Check sheet for the modelled part. Datum: model origin and axes. Units: mm. Round coordinates to 2 decimals unless told otherwise and drop trailing zeros. Loops run counter-clockwise (first coordinate to the right, second up) from the corner with the lowest first, then second, coordinate; pieces in that order, holes last. Notation, with made-up numbers: (44.25, 58.5) - (87.25, 58.5) arc R8 ccw to (87.25, 69.5) - close; hole circle Ø6 at (79, 53). An arc over 180 degrees is marked (long way). Answer in a Markdown table with one row per item. Add a question column.
(1) Cross-section at A-A on z = -25. Enter the section's corners in (x, y), then the cut area to 3 significant figures.
(2) Gauge pin test, flat end, axial feed: pin 1 (3 mm diameter, centred on x = -0.5, z = -481.5, fed in from +Y). Record the tip position at first contact, or that the pin passes through.
(3) Thickness scan on line 1 along X through (y, z) = (3.25, -240); line 2 along X through (y, z) = (6, -360); line 3 along Z through (x, y) = (-8, -3.5). Record the ranges inside material, lowest first.
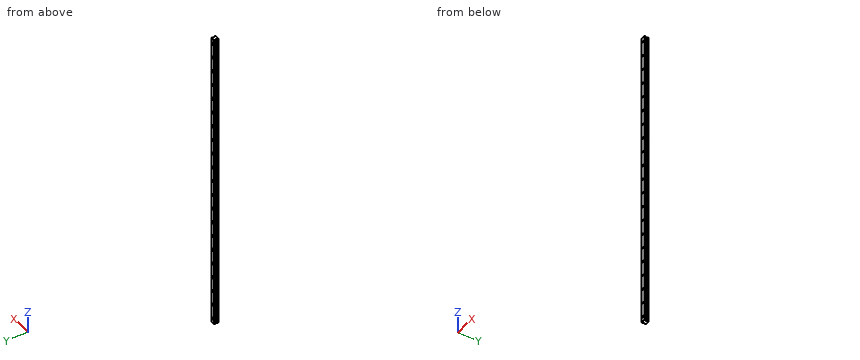
from build123d import *

# Parameters (mm, degrees)
BOSS_EXTRUDE1_DEPTH      = 620
BOSS_EXTRUDE1_DEPTH_BACK = 620
LPATTERN2_COUNT          = 21
LPATTERN2_PITCH          = 60
CHAMFER1_SIZE            = 0.5


with BuildPart() as part:
    # Sketch3 → Boss-Extrude1 (new body, two sides)
    with BuildSketch(Plane.XY) as boss_extrude1_sk:
        with BuildLine():
            Line((3, 9), (-3, 9))
            Line((-3, 9), (-7.160036564, 9))
            Line((-7.160036564, 9), (-7.767930373, 8.392105714))
            ThreePointArc((-7.767930373, 8.392105714), (-8.344874488, 7.264307267), (-9.472673258, 6.687363783))
            Line((-9.472673258, 6.687363783), (-10, 6.160037041))
            Line((-10, 6.160037041), (-10, 4.82918644))
            Line((-10, 4.82918644), (-9.472673258, 4.314376637))
            ThreePointArc((-9.472673258, 4.314376637), (-8.341068744, 3.731631743), (-7.767930373, 2.595131504))
            Line((-7.767930373, 2.595131504), (-6.550048828, 1.379235268))
            Line((-6.550048828, 1.379235268), (-6.550048828, -1.550048828))
            Line((-6.550048828, -1.550048828), (-10, -4.999922752))
            Line((-10, -4.999922752), (-10, -8))
            Line((-10, -8), (-9, -9))
            Line((-9, -9), (0, -9))
            Line((0, -9), (9, -9))
            Line((9, -9), (10, -8))
            Line((10, -8), (10, -4.999922752))
            Line((10, -4.999922752), (6.550048828, -1.550048828))
            Line((6.550048828, -1.550048828), (6.550048828, 1.379235268))
            Line((6.550048828, 1.379235268), (7.767930373, 2.595131504))
            ThreePointArc((7.767930373, 2.595131504), (8.341068744, 3.731631743), (9.472673258, 4.314376637))
            Line((9.472673258, 4.314376637), (10, 4.82918644))
            Line((10, 4.82918644), (10, 6.160037041))
            Line((10, 6.160037041), (9.472673258, 6.687363783))
            ThreePointArc((9.472673258, 6.687363783), (8.344874488, 7.264307267), (7.767930373, 8.392105714))
            Line((7.767930373, 8.392105714), (7.160036564, 9))
            Line((7.160036564, 9), (3, 9))
        make_face()
    extrude(amount=BOSS_EXTRUDE1_DEPTH)
    extrude(boss_extrude1_sk.sketch, amount=-BOSS_EXTRUDE1_DEPTH_BACK)

    # Sketch4 → Cut-Revolve1 (revolve, cut)
    with BuildSketch(Plane(origin=(0, 0, 0), x_dir=(0, 0, -1), z_dir=(1, 0, 0))):
        Polygon((-595.25, 9), (-600, 9), (-600, -9), (-597, -9), (-597, 0.5), (-595.25, 0.5), align=None)
    cut_revolve1 = revolve(axis=Axis((0, 9, 600), (0, -1, 0)), mode=Mode.SUBTRACT)

    # LPattern2: Cut-Revolve1 ×21
    with Locations(*[(0, 0, -i * LPATTERN2_PITCH) for i in range(1, LPATTERN2_COUNT)]):
        add(cut_revolve1, mode=Mode.SUBTRACT)

    # Chamfer1
    chamfer1_edges = [part.edges().sort_by_distance(p)[0] for p in [
        (-6.550048828, -0.08540678, 620),
        (-8.275024414, -3.27498579, 620),
        (-10, -6.499961376, 620),
        (-9.5, -8.5, 620),
        (0, -9, 620),
        (9.5, -8.5, 620),
        (10, -6.499961376, 620),
        (8.275024414, -3.27498579, 620),
        (6.550048828, -0.08540678, 620),
        (-8.341068744, 3.731631743, 620),
        (7.158989601, 1.987183386, 620),
        (8.341068744, 3.731631743, 620),
        (9.736336629, 4.571781538, 620),
        (-9.736336629, 4.571781538, -620),
        (-10, 5.49461174, -620),
        (10, 5.49461174, 620),
        (-9.736336629, 6.423700412, -620),
        (-7.463983469, 8.696052857, -620),
        (0, 9, -620),
        (7.463983469, 8.696052857, -620),
        (9.736336629, 6.423700412, -620),
        (10, 5.49461174, -620),
        (9.736336629, 6.423700412, 620),
        (9.736336629, 4.571781538, -620),
        (7.158989601, 1.987183386, -620),
        (6.550048828, -0.08540678, -620),
        (8.275024414, -3.27498579, -620),
        (10, -6.499961376, -620),
        (9.5, -8.5, -620),
        (0, -9, -620),
        (8.344874488, 7.264307267, 620),
        (-9.5, -8.5, -620),
        (-10, -6.499961376, -620),
        (-8.275024414, -3.27498579, -620),
        (-6.550048828, -0.08540678, -620),
        (-7.158989601, 1.987183386, -620),
        (-8.341068744, 3.731631743, -620),
        (-8.344874488, 7.264307267, -620),
        (8.344874488, 7.264307267, -620),
        (8.341068744, 3.731631743, -620),
        (7.463983469, 8.696052857, 620),
        (0, 9, 620),
        (-7.463983469, 8.696052857, 620),
        (-8.344874488, 7.264307267, 620),
        (-7.158989601, 1.987183386, 620),
        (-9.736336629, 6.423700412, 620),
        (-10, 5.49461174, 620),
        (-9.736336629, 4.571781538, 620),
    ]]
    chamfer(chamfer1_edges, length=CHAMFER1_SIZE)


solid = part.part
Answers:
| question | item | result |
|---|---|---|
| 1 | outline | (-10, -8) - (-9, -9) - (9, -9) - (10, -8) - (10, -5) - (6.55, -1.55) - (6.55, 1.38) - (7.77, 2.6) arc R2.06 cw to (9.47, 4.31) - (10, 4.83) - (10, 6.16) - (9.47, 6.69) arc R2.06 cw to (7.77, 8.39) - (7.16, 9) - (-7.16, 9) - (-7.77, 8.39) arc R2.06 cw to (-9.47, 6.69) - (-10, 6.16) - (-10, 4.83) - (-9.47, 4.31) arc R2.06 cw to (-7.77, 2.6) - (-6.55, 1.38) - (-6.55, -1.55) - (-10, -5) - close |
| 1 | area | 304 mm^2 |
| 2 | pin 1 | stops at y = 0.5 |
| 3 | line 1 | x = -7.99 to -4.75, 4.75 to 7.99 |
| 3 | line 2 | x = -10 to -4.75, 4.75 to 10 |
| 3 | line 3 | z = -619.85 to 619.85 |
